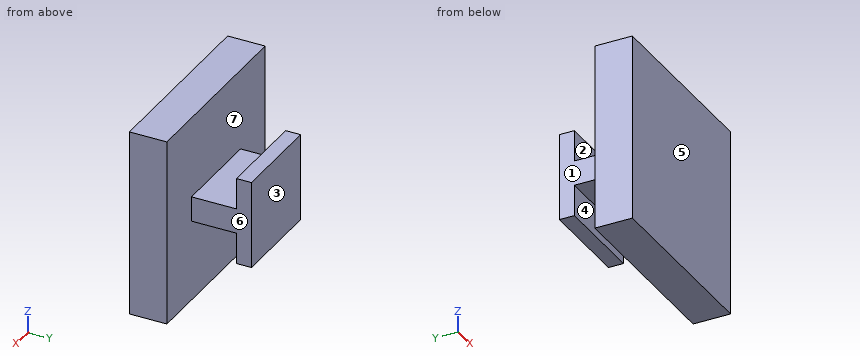
Autodesk Inventor part; units mm, degrees
ref_plane "YZ Plane" through (0, 0, 0) normal (1, 0, 0) x (0, 1, 0)
ref_plane "XZ Plane" through (0, 0, 0) normal (0, 1, 0) x (-1, 0, 0)
ref_plane "XY Plane" through (0, 0, 0) normal (0, 0, 1) x (1, 0, 0)
sketch "Sketch1" plane through (0, 0, 0) normal (0, 1, 0) x (-1, 0, 0)
  line L0 (0, 0) -> (15, 0)
  line L1 (15, 0) -> (15, 15)
  line L2 (15, 15) -> (0, 15)
  line L3 (0, 15) -> (0, 0)
  dimension "d0" = 15
  dimension "d1" = 15
extrude "Extrusion1" add sketch "Sketch1" along normal blind 3
ref_plane "Work Plane1" through (-3.75, 0, 15) normal (1, 0, 0) x (0, 0, -1)
sketch "Sketch2" plane through (-3.75, 0, 15) normal (1, 0, 0) x (0, 0, -1)
  line L0 (15, 3) -> (0, 3)
  line L1 (9.0593, 3) -> (5.9407, 3)
  line L2 (7.5, 3) -> (7.5, 8.2025)
  line L3 (0, 0) -> (0, 3)
  line L4 (7.5, 3) -> (8.5, 3)
  line L5 (8.5, 3) -> (8.5, 7.8)
  line L6 (8.5, 7.8) -> (7.5, 7.8)
  line L7 (7.5, 7.8) -> (7.5, 3)
  line L8 (8.5, 7.8) -> (11, 7.8)
  line L9 (11, 7.8) -> (11, 6.6)
  line L10 (11, 6.6) -> (8.5, 6.6)
  line L11 (8.5, 6.6) -> (8.5, 7.8)
  line L12 (6.5, 3) -> (6.5, 7.8)
  line L13 (6.5, 7.8) -> (7.5, 7.8)
  line L14 (6.5, 7.8) -> (4, 7.8)
  line L15 (4, 7.8) -> (4, 6.6)
  line L16 (4, 6.6) -> (6.5, 6.6)
  line L17 (6.5, 6.6) -> (6.5, 7.8)
  point P0 (15, 0)
  point P1 (6.5, 3)
  point P2 (8.5, 3)
  dimension "d5" = 5.2025
  dimension "d6" = 7.5
  dimension "d7" = 4.8
  dimension "d8" = 1
  dimension "d9" = 7
  dimension "d10" = 1.2
extrude "Extrusion2" add sketch "Sketch2" against normal blind 7.5
properties part number "SlangHållareFot"
Could you check a few things on this model? Use its own coordinates, in mm. Face numbers are marked on the shaded views. A direction names the side the tool comes from. Give positions to 0.01 mm unless a question says otherwise; leave off trailing zeros. Loops run counter-clockwise (first coordinate to the right, second up) from the corner with the lowest first, then second, coordinate; pieces in that order, holes last. Notation, with made-up numbers: (33.5, 87) -> (51.5, 87) arc R27 cw to (51.5, 114) -> close; hole circle Ø3 at (0, -13.75). An arc over 180 degrees is marked (long way). Put each result on its own line as item: value.
(1) For the marked faces 1, 2 and 3, which set-ups out of +Z, -Z, +X, -X, +Y, -Y let a thin tool reach every point of the face, with its end or its side?
Computed:
face 1: +Z, -Z, -X, +Y
face 2: +Z, +X, -X
face 3: +Z, -Z, +X, -X, +Y
(2) Imagine slicing it at C-C on y = 5. Write out the boundary of the cut face in (x, z), plus the area to 3 significant figures.
Computed:
outline: (-11.25, 6.5) -> (-3.75, 6.5) -> (-3.75, 8.5) -> (-11.25, 8.5) -> close
area: 15.0 mm^2
(3) Imagine slicing it at B-B on x = -6.5. Write out the boundary of the cut face in (y, z), plus the area to 3 significant figures.
Computed:
outline: (0, 0) -> (3, 0) -> (3, 6.5) -> (6.6, 6.5) -> (6.6, 4) -> (7.8, 4) -> (7.8, 11) -> (6.6, 11) -> (6.6, 8.5) -> (3, 8.5) -> (3, 15) -> (0, 15) -> close
area: 60.6 mm^2
(4) I'm going to push flat-ended pins straight in: pin 1 Ø1.3 at (x, y) = (-9, 7) entering from -Z; pin 2 Ø1.8 at (x, y) = (-6.5, 5) entering from +Z; pin 3 Ø4 at (y, z) = (5.5, 9) entering from -X; pin 4 Ø1 at (x, y) = (-13, 6.5) entering from +Z. Where does each tip first touch, or does it pass through?
Computed:
pin 1: z = 4
pin 2: z = 8.5
pin 3: x = -11.25
pin 4: through
(5) Please list where these lines run through material, in increasing order: probe 1 along Y at (x, z) = (-8, 6.25); probe 2 along X at (y, z) = (4.75, 7); probe 3 along Y at (x, z) = (-12.5, 4.25). Write a range as [from, to].
Computed:
probe 1: [0, 3], [6.6, 7.8]
probe 2: [-11.25, -3.75]
probe 3: [0, 3]
(6) Thinking about a two-plate mould opening in Y: for the marked faces 4, 5, 6 and 7, which applies, pulls with the +Y half, pulls with the -Y half, needs draft (parallel to the pull), parting line crosses it, or undercut?
Computed:
face 4: undercut
face 5: pulls with the -Y half
face 6: needs draft
face 7: undercut
(7) Imagine slicing it at D-D on z = 13. Write out the boundary of the cut face in (x, y), plus the area to 3 significant figures.
Computed:
outline: (-15, 0) -> (0, 0) -> (0, 3) -> (-15, 3) -> close
area: 45.0 mm^2
(8) Imagine slicing it at A-A on z = 10. Write out the boundary of the cut face in (x, y), plus the area to 3 significant figures.
Computed:
outline: (-15, 0) -> (0, 0) -> (0, 3) -> (-15, 3) -> close; (-11.25, 6.6) -> (-3.75, 6.6) -> (-3.75, 7.8) -> (-11.25, 7.8) -> close
area: 54.0 mm^2
